Check sheet for the drawn part. Datum: minimum x, y, z corner. Units: mm. Give positions to 0.01 mm unless a question says otherwise; leave off trailing zeros. Loops run counter-clockwise (first coordinate to the right, second up) from the corner with the lowest first, then second, coordinate; pieces in that order, holes last. Notation, with made-up numbers: (7, 79) - (19, 79) arc R19 ccw to (19, 83) - close; hole circle Ø9 at (9.25, -10). An arc over 180 degrees is marked (long way). Answer in a Markdown table with one row per item.
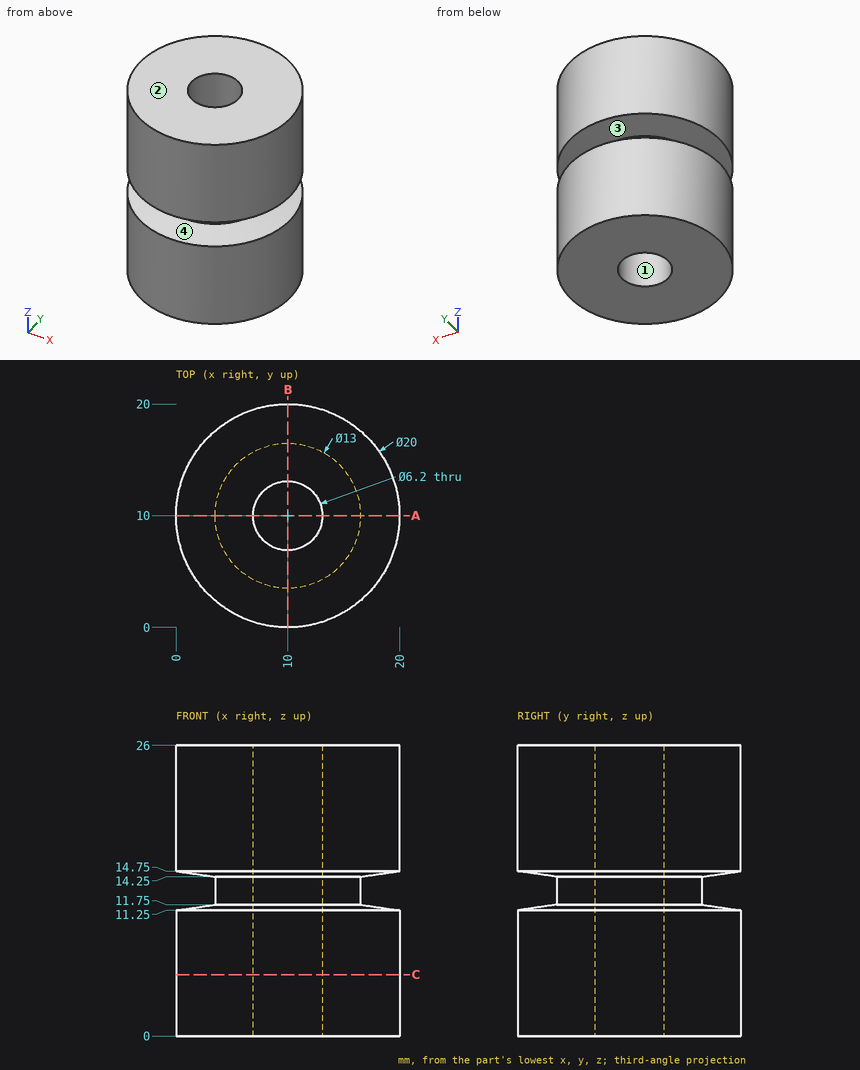
Q1. Sectioned sample at A-A (y = 10). Record the cut outline in (x, z), and give its area (3 significant figures).
Completed:
| item | result |
|---|---|
| outline | (0, 0) - (6.9, 0) - (6.9, 26) - (0, 26) - (0, 14.75) - (3.5, 14.25) - (3.5, 11.75) - (0, 11.25) - close; (13.1, 0) - (20, 0) - (20, 11.25) - (16.5, 11.75) - (16.5, 14.25) - (20, 14.75) - (20, 26) - (13.1, 26) - close |
| area | 338 mm^2 |
Q2. Draft check along Z on the marked faces 1, 2, 3 and 4. Enter one of: +Z half, -Z half, draft (parallel to the pull), parting line (faces both ways), or undercut.
Completed:
| item | result |
|---|---|
| face 1 | draft |
| face 2 | +Z half |
| face 3 | undercut |
| face 4 | undercut |
Q3. Go/stop test with flat-tipped pins: P1, Ø4, axis at x = 5, z = 10, coming from the +Y side; P2, Ø1, axis at y = 7, z = 4.5, coming from the +X side; P3, Ø4, axis at x = 14.5, y = 11.5, coming from the -Z side; P4, Ø5.5, axis at x = 10, y = 10, coming from the +Z side. Record where each tip stops, or that it passes through.
Completed:
| item | result |
|---|---|
| P1 | y = 19.54 |
| P2 | x = 19.68 |
| P3 | z = 0 |
| P4 | through |
Q4. Thickness scan on line 1 (Y direction, x = 10, z = 19); line 2 (Z direction, x = 16.5, y = 12.75); line 3 (Z direction, x = 16.5, y = 3). Record the ranges inside material, lowest first.
Completed:
| item | result |
|---|---|
| line 1 | 0 to 6.9, 13.1 to 20 |
| line 2 | 0 to 11.67, 14.33 to 26 |
| line 3 | 0 to 11.31, 14.69 to 26 |
Q5. Sectioned sample at C-C (z = 5.5). Record the cut outline in (x, y).
Completed:
| item | result |
|---|---|
| outline | circle Ø20 at (10, 10); hole circle Ø6.2 at (10, 10) |
